Answer from the drawing. Dimensions are ordinates in mm from the lowest x, y and z of the part. A direction names the side the tool comes from. Round coordinates to 2 decimals unless told otherwise and drop trailing zeros. Loops run counter-clockwise (first coordinate to the right, second up) from the corner with the lowest first, then second, coordinate; pieces in that order, holes last. Notation, with made-up numbers: M 12,-34 L 54,-34 A23 cw 54,-3 Z; hole C 54,0 d8. An arc over 180 degrees is marked long. One line per item, written item: value.
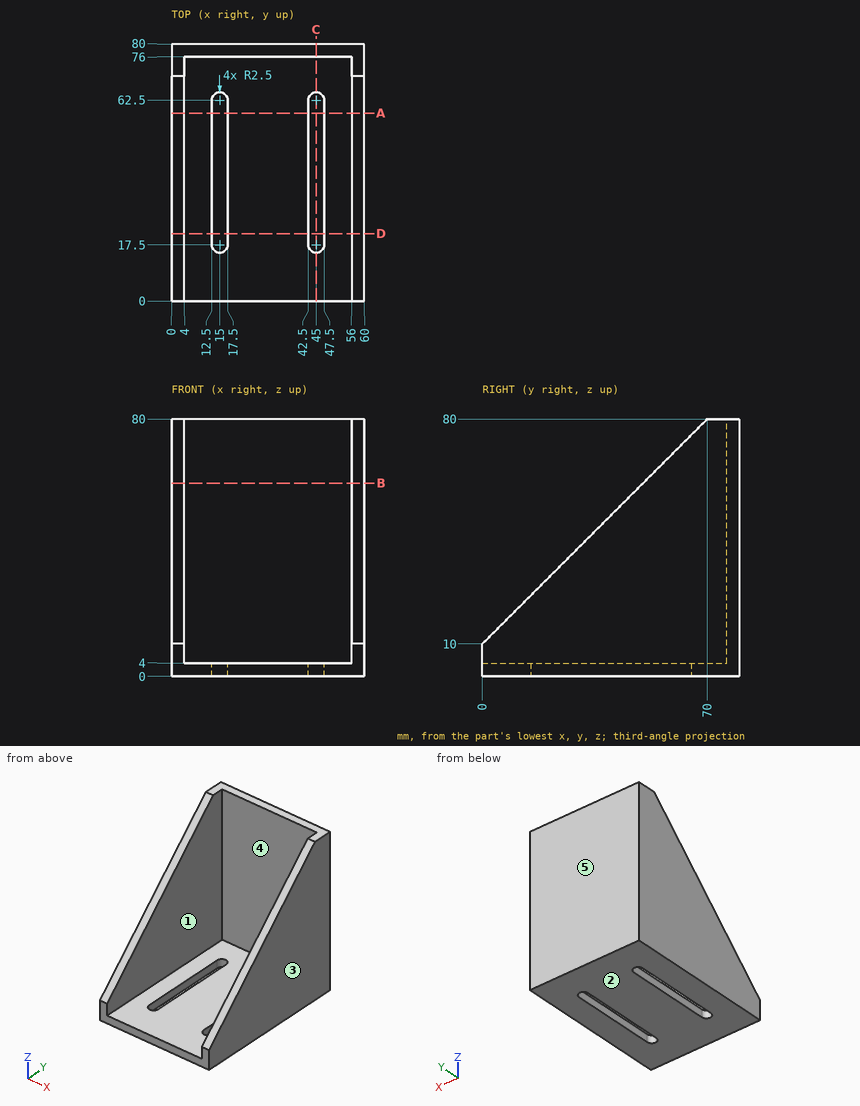
1) For the marked faces 1 and 2, determine the directions among +Z, -Z, +X, -X, +Y, -Y from which every point of the face is accessible in a straight line to the end or side of a thin tool.
Check values:
face 1: +Z, -Y
face 2: -Z, +X, -X, +Y, -Y
2) Find section D-D (y = 21). Give the vertices of the cut face in (x, z).
Check values:
outline: M 0,0 L 12.5,0 L 12.5,4 L 4,4 L 4,31 L 0,31 Z; M 17.5,0 L 42.5,0 L 42.5,4 L 17.5,4 Z; M 47.5,0 L 60,0 L 60,31 L 56,31 L 56,4 L 47.5,4 Z
3) Find section C-C (x = 45). Give the vertices of the cut face in (y, z), then the cut area to 3 significant figures.
Check values:
outline: M 0,0 L 15,0 L 15,4 L 0,4 Z; M 65,0 L 80,0 L 80,80 L 76,80 L 76,4 L 65,4 Z
area: 424 mm2
4) This flat-tipped pin is pushed along its axis until it touches: pin 1 (5 mm diameter, centred on x = 14.5, y = 31, fed in from +Z). Where does it stop, or does it pass through?
Check values:
pin 1: z = 4
5) Find section A-A (y = 58.5). Give the vertices of the cut face in (x, z), then the cut area to 3 significant figures.
Check values:
outline: M 0,0 L 12.5,0 L 12.5,4 L 4,4 L 4,68.5 L 0,68.5 Z; M 17.5,0 L 42.5,0 L 42.5,4 L 17.5,4 Z; M 47.5,0 L 60,0 L 60,68.5 L 56,68.5 L 56,4 L 47.5,4 Z
area: 716 mm2
6) Find section B-B (z = 60). Give the vertices of the cut face in (x, y).
Check values:
outline: M 0,50 L 4,50 L 4,76 L 56,76 L 56,50 L 60,50 L 60,80 L 0,80 Z
7) Find the intervals of material crossed by probe 1 along X at (y, z) = (74, 56.5); probe 2 along Z at (x, y) = (4.5, 36); probe 3 along Y at (x, z) = (14, 24), in increasing order. Write a range as from..to.
Check values:
probe 1: 0..4, 56..60
probe 2: 0..4
probe 3: 76..80
8) The mould has two halves that part along X. Classify the marked faces 3, 4 and 5: +X half, -X half, draft (parallel to the pull), parting line (faces both ways), or undercut.
Check values:
face 3: +X half
face 4: undercut
face 5: draft
